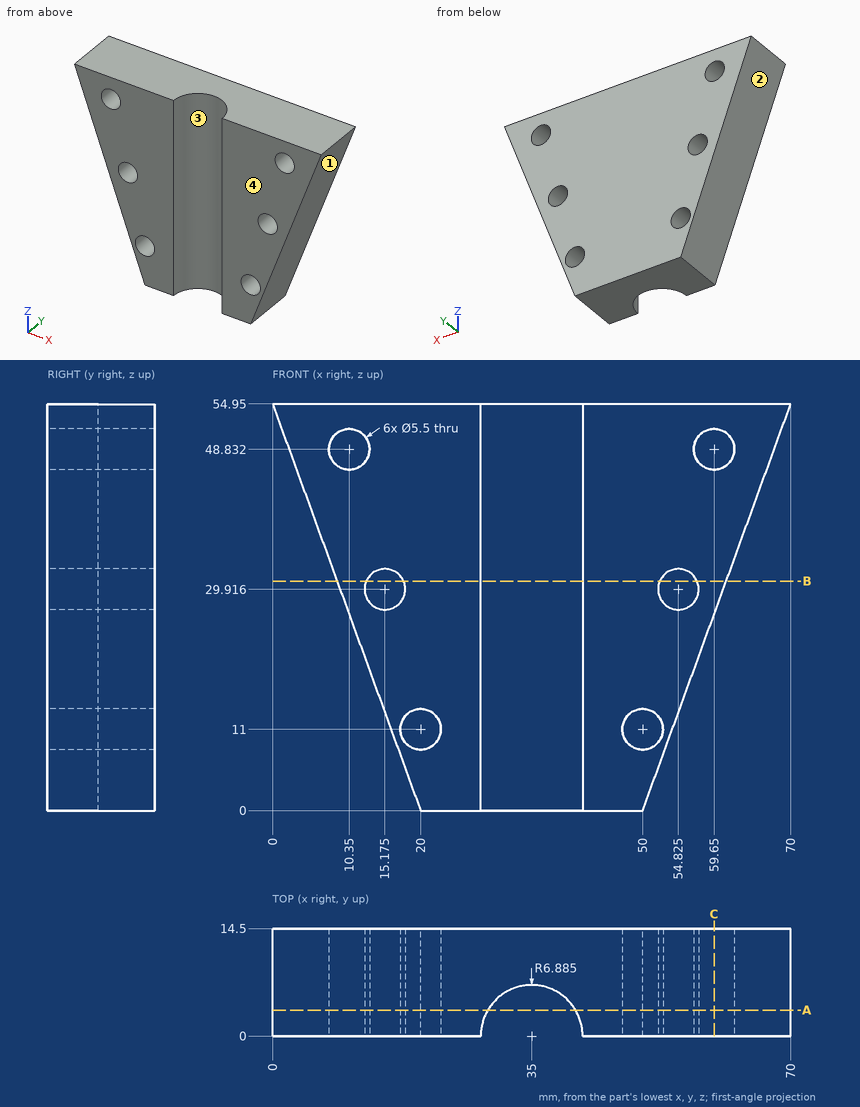
Check sheet for the drawn part. Datum: minimum x, y, z corner. Units: mm. Coordinates: 2 decimals unless noted, no trailing zeros. Order: outer loops, then holes, each group sorted by start corner. A loop starts at its lowest first (then second) coordinate and runs counter-clockwise, first axis right, second up. Notation, with made-up numbers: M -15,12 L -4,12 A16 ccw -4,29 Z; hole C 35.5,58 d8. An arc over 180 degrees is marked long. One line per question, with ' | ' between items. Start each with the question number.
Item 1: Cross-section at C-C on x = 59.65. Enter the section's corners in (y, z).
Item 2: Cross-section at A-A on y = 3.5. State how many separate pieces and enclosed holes the cut face has, then the cut area to 3 significant figures.
Item 3: Material ranges on L1, parallel to X at y = 10, z = 9.5 (1 decimal); L2, parallel to X at y = 6, z = 16.5 (1 decimal); L3, parallel to X at y = 2.75, z = 43, recorded low to high. Write a range as [from, to].
Item 4: Draft check along X on the marked faces 1, 2, 3 and 4. Enter one of: pulls with the +X half, pulls with the -X half, needs draft (parallel to the pull), parting line crosses it, or undercut.
Item 5: Cross-section at B-B on z = 31. Enter the section's corners in (x, y) (1 decimal), then the cut area to 3 significant figures.
Item 6: Gauge pin test, flat ends, axial feed: pin 1 (10 mm diameter, centred on x = 35.5, z = 29.5, fed in from -Y); pin 2 (3.5 mm diameter, centred on x = 59.65, z = 48.83, fed in from -Y); pin 3 (2 mm diameter, centred on x = 37.5, z = 40, fed in from -Y); pin 4 (1 mm diameter, centred on y = 8, z = 35.5, fed in from +X). Record the tip position at first contact, or that the pin passes through.
Findings:
1) outline: M 0,26.51 L 14.5,26.51 L 14.5,46.08 L 0,46.08 Z; M 0,51.58 L 14.5,51.58 L 14.5,54.95 L 0,54.95 Z
2) separate pieces: 2 | enclosed holes: 6 | area: 1,950 mm²
3) L1: x = [16.5, 17.7], [22.3, 47.7], [52.3, 53.5] | L2: x = [14, 31.6], [38.4, 56] | L3: x = [4.35, 28.69], [41.31, 65.65]
4) face 1: pulls with the +X half | face 2: pulls with the -X half | face 3: undercut | face 4: needs draft
5) outline: M 8.7,0 L 12.6,0 L 12.6,14.5 L 8.7,14.5 Z; M 17.7,0 L 28.1,0 A6.9 cw 41.9,0 L 52.3,0 L 52.3,14.5 L 17.7,14.5 Z; M 57.4,0 L 61.3,0 L 61.3,14.5 L 57.4,14.5 Z | area: 541 mm²
6) pin 1: stops at y = 4.14 | pin 2: passes through | pin 3: stops at y = 5.93 | pin 4: stops at x = 63.1
